```python
from build123d import *

# Parameters (mm, degrees)
IZIM2_R                               = 1.5
Y_KSEKLIK_EKSTR_ZYON1_DEPTH           = 6
Y_KSEKLIK_EKSTR_ZYON1_OTHER_WAY_DEPTH = 5
Y_KSEKLIK_EKSTR_ZYON1_OTHER_WAY_TAPER = 16
RADYUS1_R                             = 1
RADYUS2_R                             = 1
RADYUS3_R                             = 1
RADYUS4_R                             = 1
IZIM3_W                               = 1.366372993
IZIM3_H                               = 0.2
IZIM3_W_2                             = 0.2
IZIM3_H_2                             = 1.821830657
EKSTR_ZYON_NCE1_DEPTH                 = 2
IZIM4_W                               = 1.948226341
IZIM4_H                               = 3.106887173
Y_KSEKLIK_EKSTR_ZYON2_DEPTH           = 0.2
Y_KSEKLIK_EKSTR_ZYON2_DEPTH_BACK      = 0.2


with BuildPart() as part:
    # izim2 → Y_kseklik-Ekstr_zyon1 (new body)
    with BuildSketch(Plane.XY):
        with Locations((1.957696281, 2.49400279)):
            Circle(IZIM2_R)
        with Locations((1.924962477, -1.50586327)):
            Circle(IZIM2_R)
        with Locations((-2.042303717, 2.494135307)):
            Circle(IZIM2_R)
        with Locations((-2.042303717, -1.424442234)):
            Circle(IZIM2_R)
    extrude(amount=Y_KSEKLIK_EKSTR_ZYON1_DEPTH)

    # izim2 → Y_kseklik-Ekstr_zyon1 other way (add)
    with BuildSketch(Plane.XY):
        with Locations((1.957696281, 2.49400279)):
            Circle(IZIM2_R)
        with Locations((1.924962477, -1.50586327)):
            Circle(IZIM2_R)
        with Locations((-2.042303717, 2.494135307)):
            Circle(IZIM2_R)
        with Locations((-2.042303717, -1.424442234)):
            Circle(IZIM2_R)
    extrude(amount=-Y_KSEKLIK_EKSTR_ZYON1_OTHER_WAY_DEPTH, taper=Y_KSEKLIK_EKSTR_ZYON1_OTHER_WAY_TAPER)

    # Radyus1
    radyus1_edges = [part.edges().sort_by_distance(p)[0] for p in [
        (-3.542303717, 2.494135307, 0),
        (-3.542303717, 2.494135307, 6),
    ]]
    fillet(radyus1_edges, radius=RADYUS1_R)

    # Radyus2
    radyus2_edges = [part.edges().sort_by_distance(p)[0] for p in [
        (0.457696281, 2.49400279, 0),
        (0.457696281, 2.49400279, 6),
    ]]
    fillet(radyus2_edges, radius=RADYUS2_R)

    # Radyus3
    radyus3_edges = [part.edges().sort_by_distance(p)[0] for p in [
        (0.424962477, -1.50586327, 0),
        (0.424962477, -1.50586327, 6),
    ]]
    fillet(radyus3_edges, radius=RADYUS3_R)

    # Radyus4
    radyus4_edges = [part.edges().sort_by_distance(p)[0] for p in [
        (-3.542303717, -1.424442234, 0),
        (-3.542303717, -1.424442234, 6),
    ]]
    fillet(radyus4_edges, radius=RADYUS4_R)

    # izim3 → Ekstr_zyon-_nce1 (add)
    with BuildSketch(Plane.XY):
        with Locations((-0.086141829, 2.627534593)):
            Rectangle(IZIM3_W, IZIM3_H)
        with Locations((1.92848304, 0.315311653)):
            Rectangle(IZIM3_W_2, IZIM3_H_2)
        Polygon((0.748863888, -1.495674774), (-0.866926397, -1.506519004), (-0.868268648, -1.306523508), (0.747521636, -1.295679278), align=None)
        Polygon((-2.038103247, -0.248588312), (-2.059791708, 1.258759671), (-1.859812407, 1.261637071), (-1.838123947, -0.245710912), align=None)
    extrude(amount=EKSTR_ZYON_NCE1_DEPTH)

    # izim4 → Y_kseklik-Ekstr_zyon2 (add, two sides)
    with BuildSketch(Plane(origin=(0, 0, 0), x_dir=(0, 0, -1), z_dir=(1, 0, 0))) as y_kseklik_ekstr_zyon2_sk:
        with Locations((-1.005175918, 4.148063822)):
            Rectangle(IZIM4_W, IZIM4_H)
    extrude(amount=Y_KSEKLIK_EKSTR_ZYON2_DEPTH)
    extrude(y_kseklik_ekstr_zyon2_sk.sketch, amount=-Y_KSEKLIK_EKSTR_ZYON2_DEPTH_BACK)


solid = part.part
```
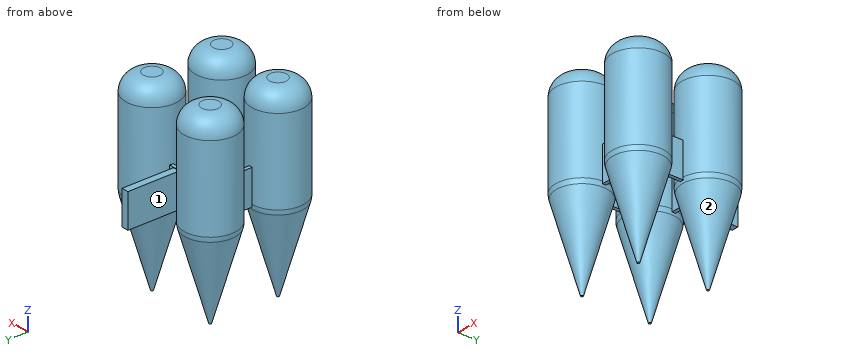
Check sheet for the modelled part. Datum: model origin and axes. Units: mm. Face numbers are marked on the shaded views. A direction names the side the tool comes from. Coordinates: 2 decimals unless noted, no trailing zeros. Loops run counter-clockwise (first coordinate to the right, second up) from the corner with the lowest first, then second, coordinate; pieces in that order, holes last. Notation, with made-up numbers: M 36.5,65.25 L 45.5,65.25 A20 ccw 45.5,95.25 Z; hole C 42,62.25 d6. An arc over 180 degrees is marked long. Answer as a JSON object with one key per item and string values.
1. Depth check by flat-ended pin: P1, Ø1.6, axis at y = 5, z = 1.5, coming from the -X side; P2, Ø0.8, axis at y = 0.5, z = 1, coming from the +X side; P3, Ø4, axis at y = -1.5, z = -2.5, coming from the +X side. Enter the tip coordinate at first touch or a pass-through.
Outcome:
{"P1": "x = -0.2", "P2": "x = 2.03", "P3": "x = 3.28"}
2. Scan lines: L1, parallel to X at y = 3.25, z = 0.5; L2, parallel to X at y = -1, z = 5; L3, parallel to X at y = 3.5, z = 4.25. Record each from-to range of solid material in increasing order. Write a range as from..to.
Outcome:
{"L1": "-3.34..-0.75, -0.2..0.2, 0.66..3.25", "L2": "-3.48..-0.6, 0.51..3.34", "L3": "-3.16..-0.93, 0.85..3.07"}
3. Sectioned sample at B-B on z = 1.25. Record the cut outline in (x, y).
Outcome:
{"outline": "M -2.06,0.99 L -2.04,0.08 A1.5 ccw long -0.54,-1.5 L 0.42,-1.5 A1.5 ccw long 2.03,-0.01 L 2.03,1 A1.5 ccw long 0.48,2.73 L 0.2,2.73 L 0.2,5.7 L -0.2,5.7 L -0.2,2.73 L -0.56,2.73 A1.5 ccw long Z; hole M -1.86,1.01 L -1.84,0.06 A1.5 cw -0.55,-1.3 L 0.44,-1.3 A1.5 cw 1.83,-0.01 L 1.83,1 A1.5 cw 0.46,2.53 L -0.54,2.53 A1.5 cw Z"}
4. Sectioned sample at C-C on y = 3.75. Count the separate pieces of the cut face and the enclosed holes in it, and give its area (3 significant figures).
Outcome:
{"separate pieces": "3", "enclosed holes": "0", "area": "20.7 mm²"}
5. Sectioned sample at D-D on z = 4. Record the cut outline in (x, y).
Outcome:
{"outline": "C -2.04,-1.42 d3; C -2.04,2.49 d3; C 1.92,-1.51 d3; C 1.96,2.49 d3"}
6. Access from +Z, -Z, +X, -X, +Y, -Y to the whole of each face (thin tool, end or side, straight path). Record for the marked faces 1 and 2.
Outcome:
{"face 1": "+Z, -Z, +Y", "face 2": "-Z"}
